Autodesk Inventor part; units mm, degrees
ref_plane "YZ Plane" through (0, 0, 0) normal (1, 0, 0) x (0, 1, 0)
ref_plane "XZ Plane" through (0, 0, 0) normal (0, 1, 0) x (-1, 0, 0)
ref_plane "XY Plane" through (0, 0, 0) normal (0, 0, 1) x (1, 0, 0)
sketch "Boceto1" plane through (0, 0, 0) normal (0, 1, 0) x (-1, 0, 0)
  line L0 (0, 0) -> (-15, 0)
  line L1 (0, 0) -> (7.0223, -1.8816)
  line L2 (0, 0) -> (7.27, 0) construction
  line L3 (8.8653, -2.3754) -> (7.0223, -1.8816)
  line L4 (8.8653, -2.3754) -> (3.6889, -21.694)
  line L5 (8.8653, -2.3754) -> (28.8653, -2.3754) construction
  line L6 (-15, 0) -> (-15, -3)
  line L7 (-15, -3) -> (0, -3)
  line L8 (0, -3) -> (5.2175, -4.398)
  line L9 (5.2175, -4.398) -> (25.2175, -4.398) construction
  line L10 (3.6889, -21.694) -> (0.7911, -20.9175)
  line L11 (0.7911, -20.9175) -> (5.2175, -4.398)
  point P0 (4.2275, -19.6837)
  dimension "d0" = 15
  dimension "d1" = 7.27
  dimension "d2" = 15
  dimension "d3" = 1.908
  dimension "d4" = 20
  dimension "d5" = 105
  dimension "d7" = 3
extrude "Extrusión1" add sketch "Boceto1" along normal blind 22
sketch "Boceto2" plane through (0, 0, 0) normal (-0.258819, 0, 0.9659258) x (0.9659258, 0, 0.258819)
  line L0 (-9.178, 0) -> (-9.178, 22)
  line L1 (-9.178, 0) -> (-9.178, 9)
  line L2 (-9.178, 9) -> (0, 9)
  line L3 (0, 9) -> (0, 13)
  line L4 (0, 13) -> (-9.178, 13)
  line L5 (-9.178, 13) -> (-9.178, 9)
  line L6 (0, 0) -> (0, 11)
  line L7 (0, 0) -> (0, 22)
  point P0 (-9.178, 13)
  dimension "d12" = 9
  dimension "d13" = 4
  dimension "d53" = 11
extrude "Extrusión2" cut sketch "Boceto2" against normal blind 1
sketch "Boceto3" plane through (0, 0, 0) normal (0, 0, 1) x (1, 0, 0)
  line L0 (15, 0) -> (15, 22)
  line L1 (15, 7) -> (15, 3.2945)
  line L2 (15, 3.2945) -> (15, 3)
  line L3 (15, 22) -> (0, 22)
  line L4 (15, 22) -> (15, 11)
  line L5 (15, 0) -> (15, 22)
  line L6 (0, 0) -> (0, 22)
  line L7 (13.0524, 11) -> (13.0524, 9)
  line L8 (13.0524, 9) -> (15, 9)
  line L9 (0, 9) -> (15, 9)
  line L10 (15, 11) -> (15, 13)
  line L11 (15, 13) -> (0, 13)
  point P0 (0, 9)
  point P1 (0, 13)
  dimension "d48" = 11
  dimension "d49" = 2
  dimension "d50" = 2
sketch "Boceto7" plane through (-3.6889, 0, -21.694) normal (-0.9659258, 0, -0.258819) x (-0.258819, 0, 0.9659258)
  line L0 (0, 0) -> (0, 22)
  line L1 (0, 0) -> (0, 3)
  line L2 (0, 3) -> (20, 3)
  line L3 (20, 3) -> (20, 19)
  line L4 (20, 13) -> (20, 22)
  line L5 (20, 19) -> (17, 19)
  line L6 (17, 19) -> (17.1022, 3)
  line L7 (17.1022, 0) -> (17.1022, 22)
  line L8 (17, 19) -> (0, 19)
  line L9 (0, 22) -> (3, 22)
  line L10 (17.1022, 22) -> (0, 22)
  line L11 (3, 22) -> (3, 0)
  point P0 (20, 0)
  point P1 (20, 7)
  point P2 (3, 19)
  point P3 (3, 3)
  dimension "d30" = 3
  dimension "d31" = 16
  dimension "d32" = 3
  dimension "d33" = 3
extrude "Extrusión6" add sketch "Boceto7" along normal blind 2 contours L11 L8 L6 L2
fillet "Empalme1" radius 1 4 edges at (-6.3972, 11, -19.3138) (-8.2222, 3, -12.503) (-10.0339, 11, -5.7415) (-8.2089, 19, -12.5523)
sketch "Boceto8" plane through (-3.6889, 0, -21.694) normal (-0.9659258, 0, -0.258819) x (-0.258819, 0, 0.9659258)
  line L0 (0, 0) -> (20, 0)
  line L1 (0, 0) -> (0, 1.5)
  line L2 (0, 0) -> (0, 22)
  line L3 (0, 1.5) -> (1.5, 1.5)
  line L4 (1.5, 1.5) -> (1.5, 20.5)
  line L5 (1.5, 20.5) -> (19, 20.5)
  line L6 (20, 13) -> (20, 22)
  line L7 (19, 20.5) -> (19, 1.5)
  line L8 (19, 1.5) -> (1.5, 1.5)
  circle A0 centre (1.5, 1.5) radius 0.75
  circle A1 centre (1.5, 20.5) radius 0.75
  circle A2 centre (19, 20.5) radius 0.75
  circle A3 centre (19, 1.5) radius 0.75
  dimension "d37" = 1.5
  dimension "d38" = 1.5
  dimension "d39" = 19
  dimension "d40" = 17.5
  dimension "d41" = 19
  dimension "d42" = 1.5
  dimension "d43" = 1.5
  dimension "d44" = 1.5
  dimension "d45" = 1.5
extrude "Extrusión7" add sketch "Boceto8" along normal blind 2 contours A0 L4 L3 | L3 L8 A0 | L4 A0 L8 | A1 L5 L4 | L4 L5 A1 | A3 L7 L8 | L8 L7 A3 | A2 L7 L5 | L5 L7 A2
extrude "Extrusión8" cut sketch "Boceto3" against normal blind 1 contours L8 L9 L6 L11 L0
sketch "Boceto9" plane through (15, 0, 0) normal (1, 0, 0) x (0, 0, -1)
  line L0 (0, 13) -> (0, 11)
  circle A0 centre (0, 11) radius 3
  circle A1 centre (0, 11) radius 2
  line L1 (0, 15.8082) -> (0, 4.1439)
  point P0 (0, 0)
  point P1 (0, 9)
  point P2 (0, 8)
  point P3 (0, 14)
  dimension "d54" = 2
  dimension "d55" = 4
extrude "Extrusión9" add sketch "Boceto9" along normal blind 20 contours L1 A0 A1 picked at (2.6416, 11.2225)
properties part number "GY_906 Casetop"
The listing builds one solid part. Answer for the finished solid, in the listing's coordinates (mm). A direction names the side the tool comes from. Coordinates: 2 decimals unless noted, no trailing zeros. Write each loop counter-clockwise with the first axis right and the second up, starting at its lowest first coordinate (ties: lowest second). Pieces come first, ordered by that corner, then holes. Notation, with made-up numbers: M 56,-10.5 L 80,-10.5 A36 ccw 80,28.5 Z; hole C -17,74.25 d9. An arc over 180 degrees is marked long. Use a Markdown table: item, result. Add a question column.
1. For a pull along Y with two mould halves and no side action, classify faces 5 (the flat face through (-2.26, 10.85, -21.31)), 6 (the flat face through (-7, 3, -12)), 7 (the flat face through (3, 13, -0.8)) as +Y half, -Y half, draft (parallel to the pull), parting line (faces both ways), or undercut.
2. Straight lines are drawn through the part: line 1 along Z through (x, y) = (2, 15.5); line 2 along Y through (x, z) = (-2, -0.75); line 3 along Z through (x, y) = (13, 11). For each, find the intervals that lie inside material, in ascending order. Write a range as [from, to].
3. Section B-B (x = 19.5) is taken. Give the vertices of the cut face in (y, z).
4. Which of the six approach directions +Z, -Z, +X, -X, +Y, -Y give full straight-line access (tool end or side, diameter ignored) to faces 1 (the flat face through (7, 11, -1)), 2 (the cylindrical face through (-7.9, 18.7, -12.6)), 3 (the cylindrical face through (25, 11, -2)), 4 (the cylindrical face through (25, 11, -3))?
5. Given P1, Ø2.5, axis at y = 19, z = -2, coming from the +X side; P2, Ø2, axis at y = 10, z = -18, coming from the -X side; P3, Ø6, axis at x = 13.5, y = 12.5, coming from the -Z side, each flat-ended and moving along its own axis, determine where each tip first touches the part or whether it passes through.
6. Section A-A (x = -1.5) is taken. Give the vertices of the cut face in (y, z).
Data:
| question | item | result |
|---|---|---|
| 1 | face 5 | draft |
| 1 | face 6 | -Y half |
| 1 | face 7 | undercut |
| 2 | line 1 | z = [-3, 0] |
| 2 | line 2 | y = [0, 9], [13, 22] |
| 2 | line 3 | z = [-3, -1] |
| 3 | outline | M 8,0 A3 ccw 14,0 L 13,0 A2 cw 9,0 Z |
| 4 | face 1 | +Z, -X |
| 4 | face 2 | -Z, -X, +Y |
| 4 | face 3 | +Z, +X |
| 4 | face 4 | -Z, +X |
| 5 | P1 | stops at x = 15 |
| 5 | P2 | stops at x = -7.02 |
| 5 | P3 | stops at z = -3 |
| 6 | outline | M 0,-21.11 L 22,-21.11 L 22,-18.27 L 0,-18.27 Z; M 0,-3.4 L 22,-3.4 L 22,-0.4 L 13,-0.4 L 13,-1.44 L 9,-1.44 L 9,-0.4 L 0,-0.4 Z |
